Part model, mm, in its own coordinate system. Round coordinates to 2 decimals unless told otherwise and drop trailing zeros. Loops run counter-clockwise (first coordinate to the right, second up) from the corner with the lowest first, then second, coordinate; pieces in that order, holes last. Notation, with made-up numbers: (-39.5, -23.5) -> (-25.5, -23.5) arc R13 ccw to (-25.5, -15.5) -> close; hole circle Ø11 at (-39, 76.25). An arc over 180 degrees is marked (long way). Answer as CSV lines item,"result".
from build123d import *

# Parameters (mm, degrees)
F0_R     = 27.051
F0_R_2   = 6.35
F1_DEPTH = 0.381
F2_D     = 2.9464
F3_D     = 2.1844


with BuildPart() as f1:
    # F0 (on Top) → F1 (new body)
    with BuildSketch(Plane.XY):
        Circle(F0_R)
        Circle(F0_R_2, mode=Mode.SUBTRACT)
    extrude(amount=F1_DEPTH)

    # F2 (through all)
    with Locations(Plane(origin=(0, 0, 0), x_dir=(1, 0, 0), z_dir=(0, 0, -1))):
        with Locations((-21.7678, -12.573), (-12.573, -21.7678), (12.573, -21.7678), (21.7678, -12.573), (21.7678, 12.573), (12.573, 21.7678), (-12.573, 21.7678), (-21.7678, 12.573)):
            Hole(F2_D / 2)

    # F3 (through all)
    with Locations(Plane(origin=(0, 0, 0), x_dir=(1, 0, 0), z_dir=(0, 0, -1))):
        with Locations((0, 9.398), (8.128, 4.699), (-8.1389067448, -4.699), (0, 0), (0.0054533724, -9.388554482), (8.1389067448, -4.699), (-8.1334533724, 4.689554482)):
            Hole(F3_D / 2)


solid = f1.part
Q1. Saw through at C-C, the plane x = -8.5. Write the cut outline in (y, z), then the cut area to 3 significant figures.
Geometry results:
outline,"(-25.68, 0) -> (-5.72, 0) -> (-5.72, 0.38) -> (-25.68, 0.38) -> close; (-3.66, 0) -> (3.67, 0) -> (3.67, 0.38) -> (-3.66, 0.38) -> close; (5.73, 0) -> (25.68, 0) -> (25.68, 0.38) -> (5.73, 0.38) -> close"
area,"18.0 mm2"
Q2. Drill centre lines: line 1 along X through (y, z) = (5, 0.1); line 2 along Y through (x, z) = (-21.5, 0.3); line 3 along X through (y, z) = (-4, 0.25). Where is each one in solid material? Low to high.
Geometry results:
line 1,"-26.58 to -9.19, -7.09 to -3.91, 3.91 to 7.09, 9.19 to 26.58"
line 2,"-16.42 to -14.02, -11.12 to 11.12, 14.02 to 16.42"
line 3,"-26.75 to -8.98, -7.29 to -4.93, 4.93 to 7.29, 8.97 to 26.75"
Q3. Drop a flat-ended pin along its axis: P1, Ø2.5, axis at x = -12.57, y = -21.77, coming from the -Z side (1 decimal). Give the stop position or say it passes through.
Geometry results:
P1,"through"
Q4. Saw through at D-D, the plane z = 0.2. Give the number of separate pieces and of enclosed holes in the cut face, then the cut area to 3 significant figures.
Geometry results:
separate pieces,"1"
enclosed holes,"15"
area,"2,100 mm2"
Q5. Saw through at B-B, the plane x = 0. Write the cut outline in (y, z).
Geometry results:
outline,"(-27.05, 0) -> (-10.49, 0) -> (-10.49, 0.38) -> (-27.05, 0.38) -> close; (-8.31, 0) -> (-6.35, 0) -> (-6.35, 0.38) -> (-8.31, 0.38) -> close; (6.35, 0) -> (8.3, 0) -> (8.3, 0.38) -> (6.35, 0.38) -> close; (10.48, 0) -> (27.05, 0) -> (27.05, 0.38) -> (10.48, 0.38) -> close"
Q6. Two-plate mould, pull along Y, no slides. Class faces 1 (the face through (25.8, 8.13, 0.19)), 2 (the face through (0.242, 10.455, 0.193)), 3 (the face through (6, -6, 0)): pulls with the +Y half, pulls with the -Y half, needs draft (parallel to the pull), parting line crosses it, or undercut.
Geometry results:
face 1,"parting line crosses it"
face 2,"undercut"
face 3,"needs draft"
Q7. Saw through at A-A, the plane y = 0. Write the cut outline in (x, z), then the cut area to 3 significant figures.
Geometry results:
outline,"(-27.05, 0) -> (-6.35, 0) -> (-6.35, 0.38) -> (-27.05, 0.38) -> close; (6.35, 0) -> (27.05, 0) -> (27.05, 0.38) -> (6.35, 0.38) -> close"
area,"15.8 mm2"
